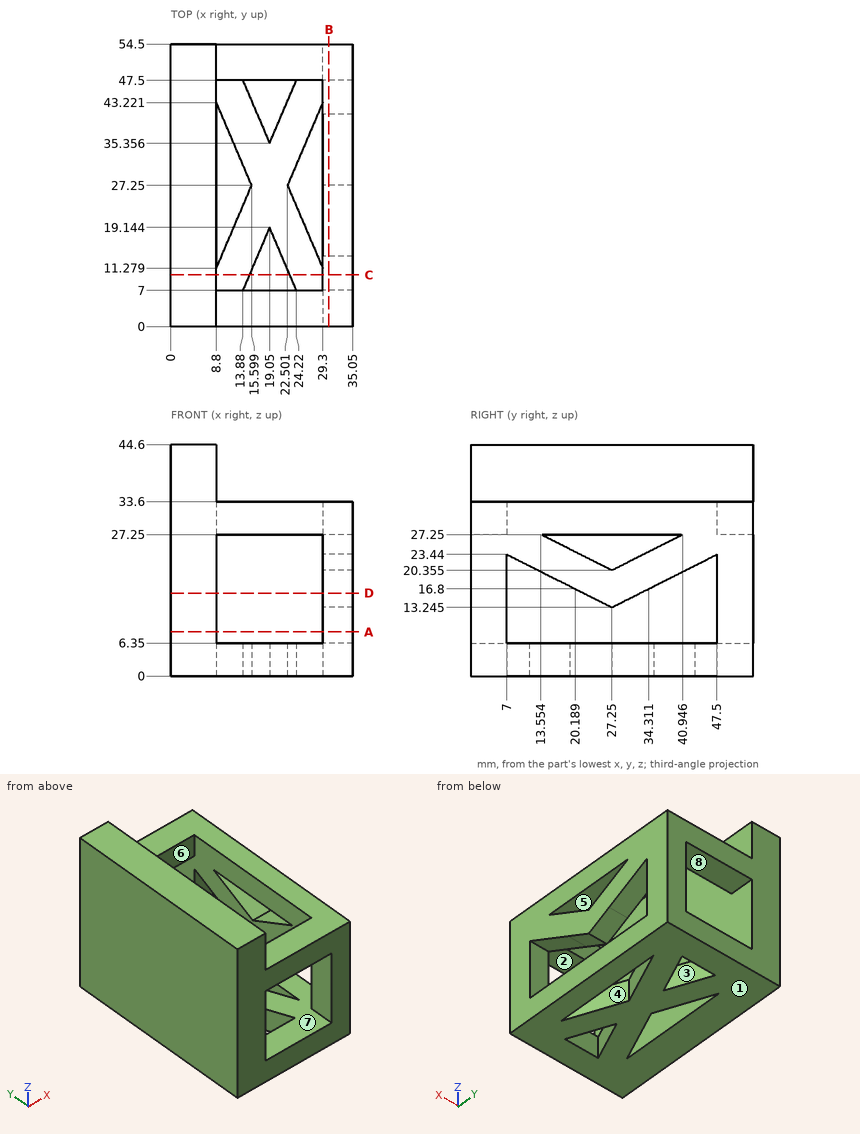
Check sheet for the drawn part. Datum: minimum x, y, z corner. Units: mm. A direction names the side the tool comes from. Round coordinates to 2 decimals unless told otherwise and drop trailing zeros. Loops run counter-clockwise (first coordinate to the right, second up) from the corner with the lowest first, then second, coordinate; pieces in that order, holes last. Notation, with made-up numbers: (6.25, -1.75) - (64.25, -1.75) arc R11 cw to (64.25, 18.25) - close; hole circle Ø1 at (-22, 38.25). An arc over 180 degrees is marked (long way). Answer as a JSON object with one key per item and string values. Group by question number.
Q1. Sectioned sample at B-B, the plane x = 30.5. Count the separate pieces of the cut face and the enclosed holes in it, plus the area to 3 significant figures.
Q2. Sectioned sample at D-D, the plane z = 16. Enter the section's corners in (x, y), plus the area to 3 significant figures.
Q3. Gauge pin test, flat ends, axial feed: P1, Ø5, axis at x = 25, z = 19, coming from the +Y side; P2, Ø3, axis at y = 40.5, z = 6.5, coming from the +X side. Record the tip position at first contact, or that the pin passes through.
Q4. Scan lines: line 1 along Z through (x, y) = (18.5, 48.5); line 2 along Y through (x, z) = (16.5, 30); line 3 along X through (y, z) = (25.5, 12). Record each from-to range of solid material in increasing order. Write a range as [from, to].
Q5. Sectioned sample at A-A, the plane z = 8.5. Enter the section's corners in (x, y).
Q6. Set-up check for the marked faces 4, 5, 6, 7 and 8: record each of +Z, -Z, +X, -X, +Y, -Y from which the full face is reachable in a straight line by a thin tool's end or side.
Q7. Sectioned sample at C-C, the plane y = 10. Enter the section's corners in (x, z), plus the area to 3 significant figures.
Q8. Mould release check, pull along Z, two halves, no side actions. Record for the marked faces 1, 2 and 3: released by +Z, released by -Z, zero draft, split by the parting line, or undercut.
Solution:
{
 "1": {"separate pieces": "1", "enclosed holes": "2", "area": "1,250 mm²"},
 "2": {"outline": "(0, 0) - (8.8, 0) - (8.8, 54.5) - (0, 54.5) - close; (29.3, 0) - (35.05, 0) - (35.05, 7) - (29.3, 7) - close; (29.3, 21.78) - (35.05, 21.78) - (35.05, 32.72) - (29.3, 32.72) - close; (29.3, 47.5) - (35.05, 47.5) - (35.05, 54.5) - (29.3, 54.5) - close", "area": "623 mm²"},
 "3": {"P1": "passes through", "P2": "stops at x = 35.05"},
 "4": {"line 1": "z = [0, 6.35], [27.25, 33.6]", "line 2": "y = [0, 7], [47.5, 54.5]", "line 3": "x = [0, 8.8]"},
 "5": {"outline": "(0, 0) - (8.8, 0) - (8.8, 54.5) - (0, 54.5) - close; (29.3, 0) - (35.05, 0) - (35.05, 7) - (29.3, 7) - close; (29.3, 47.5) - (35.05, 47.5) - (35.05, 54.5) - (29.3, 54.5) - close"},
 "6": {"face 4": "+Z, -Z", "face 5": "+X", "face 6": "+Z", "face 7": "none", "face 8": "+Y, -Y"},
 "7": {"outline": "(0, 0) - (15.16, 0) - (15.16, 6.35) - (8.8, 6.35) - (8.8, 44.6) - (0, 44.6) - close; (22.94, 0) - (35.05, 0) - (35.05, 6.35) - (22.94, 6.35) - close; (29.3, 21.93) - (35.05, 21.93) - (35.05, 33.6) - (29.3, 33.6) - close", "area": "577 mm²"},
 "8": {"face 1": "released by -Z", "face 2": "undercut", "face 3": "zero draft"}
}
